CAD build for the part. Positions are in the model's coordinates, mm. A direction names the side the tool comes from. Give positions to 0.01 mm unless a question says otherwise; leave off trailing zeros. Write each loop counter-clockwise with the first axis right and the second up, starting at its lowest first coordinate (ties: lowest second). Pieces come first, ordered by that corner, then holes. Notation, with made-up numbers: (4.25, 9.5) -> (50.25, 9.5) arc R20 cw to (50.25, 27.5) -> close; hole circle Ø4 at (16, 30). An arc over 180 degrees is marked (long way). Answer as a JSON object with one key per item and string values.
```python
from build123d import *

# Parameters (mm, degrees)
SKETCH_1_W          = 16.2
SKETCH_1_H          = 5.8
EXTRUDE_1_DEPTH     = 10
SKETCH_2_W          = 15.2
SKETCH_2_H          = 4.8
CUT_EXTRUDE_1_DEPTH = 6
SKETCH_3_R          = 0.5
EXTRUDE_2_DEPTH     = 6
SKETCH_4_W          = 0.5
SKETCH_4_H          = 0.5
CUT_EXTRUDE_2_DEPTH = 5


with BuildPart() as part:
    # Эскиз1 → Бобышка-Вытянуть1 (new body)
    with BuildSketch(Plane(origin=(0, 0, 0), x_dir=(1, 0, 0), z_dir=(0, 1, 0))):
        Rectangle(SKETCH_1_W, SKETCH_1_H)
    extrude(amount=EXTRUDE_1_DEPTH)

    # Эскиз2 → Вырез-Вытянуть1 (cut)
    with BuildSketch(Plane(origin=(0, 10, 0), x_dir=(1, 0, 0), z_dir=(0, 1, 0))):
        Rectangle(SKETCH_2_W, SKETCH_2_H)
    extrude(amount=-CUT_EXTRUDE_1_DEPTH, mode=Mode.SUBTRACT)

    # Эскиз3 → Бобышка-Вытянуть2 (add)
    with BuildSketch(Plane(origin=(0, 4, 0), x_dir=(1, 0, 0), z_dir=(0, 1, 0))):
        with Locations(Location((-4.6, 0, 0), (0, 0, 270))):
            Circle(SKETCH_3_R)
        with Locations(Location((-1.6, 0, 0), (0, 0, 270))):
            Circle(SKETCH_3_R)
        with Locations(Location((1.6, 0, 0), (0, 0, 270))):
            Circle(SKETCH_3_R)
        with Locations(Location((4.6, 0, 0), (0, 0, 270))):
            Circle(SKETCH_3_R)
    extrude(amount=EXTRUDE_2_DEPTH)

    # Эскиз4 → Вырез-Вытянуть2 (cut)
    with BuildSketch(Plane(origin=(0, 10, 0), x_dir=(1, 0, 0), z_dir=(0, 1, 0))):
        with Locations((-6.35, 2.65)):
            Rectangle(SKETCH_4_W, SKETCH_4_H)
        with Locations((-7.85, 1.15)):
            Rectangle(SKETCH_4_W, SKETCH_4_H)
    cut_extrude_2 = extrude(amount=-CUT_EXTRUDE_2_DEPTH, mode=Mode.SUBTRACT)

    # Зеркальное отражение1: Вырез-Вытянуть2 across plane
    add(cut_extrude_2.mirror(Plane(origin=(0, 0, 0), x_dir=(0, 0, 1), z_dir=(1, 0, 0))), mode=Mode.SUBTRACT)


solid = part.part
```
1) Slice it at C-C (z = 0). List the corners of the cut face in (x, y), then the cut area to 3 significant figures.
Model answer:
{"outline": "(-8.1, 0) -> (8.1, 0) -> (8.1, 10) -> (7.6, 10) -> (7.6, 4) -> (5.1, 4) -> (5.1, 10) -> (4.1, 10) -> (4.1, 4) -> (2.1, 4) -> (2.1, 10) -> (1.1, 10) -> (1.1, 4) -> (-1.1, 4) -> (-1.1, 10) -> (-2.1, 10) -> (-2.1, 4) -> (-4.1, 4) -> (-4.1, 10) -> (-5.1, 10) -> (-5.1, 4) -> (-7.6, 4) -> (-7.6, 10) -> (-8.1, 10) -> close", "area": "94.8 mm2"}
2) Slice it at A-A (y = 6). List the corners of the cut face in (x, z), then the cut area to 3 significant figures.
Model answer:
{"outline": "(-8.1, -2.9) -> (-6.6, -2.9) -> (-6.6, -2.4) -> (-7.6, -2.4) -> (-7.6, -1.4) -> (-8.1, -1.4) -> close; (-8.1, -0.9) -> (-7.6, -0.9) -> (-7.6, 2.4) -> (7.6, 2.4) -> (7.6, -0.9) -> (8.1, -0.9) -> (8.1, 2.9) -> (-8.1, 2.9) -> close; (-6.1, -2.9) -> (6.1, -2.9) -> (6.1, -2.4) -> (-6.1, -2.4) -> close; circle Ø1 at (-4.6, 0); circle Ø1 at (-1.6, 0); circle Ø1 at (1.6, 0); circle Ø1 at (4.6, 0); (6.6, -2.9) -> (8.1, -2.9) -> (8.1, -1.4) -> (7.6, -1.4) -> (7.6, -2.4) -> (6.6, -2.4) -> close", "area": "23.1 mm2"}
3) 3-axis set-ups, long thin cutter, end or side, ignore diameter. For faces 1 (the flat face through (1.6, 10, 0)), 2 (the cylindrical face through (-2.088, 6.958, -0.108)): which of +Z, -Z, +X, -X, +Y, -Y reach the whole face in a straight line?
Model answer:
{"face 1": "+Z, -Z, +X, -X, +Y", "face 2": "+Y"}
4) Slice it at B-B (x = -0.5). List the corners of the cut face in (y, z).
Model answer:
{"outline": "(0, -2.9) -> (10, -2.9) -> (10, -2.4) -> (4, -2.4) -> (4, 2.4) -> (10, 2.4) -> (10, 2.9) -> (0, 2.9) -> close"}
5) Wall check: probe 1 along Z at (x, y) = (5, 8); probe 2 along X at (y, z) = (6.75, -2.2); probe 3 along Z at (x, y) = (5.5, 6.5). Give the ranges that are in metal, low to high.
Model answer:
{"probe 1": "z = -2.9 to -2.4, -0.3 to 0.3, 2.4 to 2.9", "probe 2": "x = -8.1 to -7.6, 7.6 to 8.1", "probe 3": "z = -2.9 to -2.4, 2.4 to 2.9"}
6) Pin check, flat tip, straight feed: pin 1 (0.6 mm diameter, centred on x = 8, z = -1, fed in from +Y). Stop position of the tip, or through.
Model answer:
{"pin 1": "stops at y = 10"}
7) Mould opens along X. For faces 3 (the flat face through (-7.6, 7, 0)), 4 (the flat face through (8.1, 5, 0)), 5 (the flat face through (-4.6, 10, 0)) say: released by +X, released by -X, zero draft, split by the parting line, or undercut.
Model answer:
{"face 3": "undercut", "face 4": "released by +X", "face 5": "zero draft"}
8) Slice it at D-D (z = 2). List the corners of the cut face in (x, y).
Model answer:
{"outline": "(-8.1, 0) -> (8.1, 0) -> (8.1, 10) -> (7.6, 10) -> (7.6, 4) -> (-7.6, 4) -> (-7.6, 10) -> (-8.1, 10) -> close"}
